The model under review builds one solid part; all positions refer to its coordinate system, in mm. A direction names the side the tool comes from. Round coordinates to 2 decimals unless told otherwise and drop trailing zeros. Write each loop counter-clockwise with the first axis right and the second up, starting at its lowest first coordinate (ties: lowest second). Pieces come first, ordered by that corner, then holes.
Item 1: Draft analysis for pull direction Y (two halves, no side actions). For faces 1 (the face through (-68.862, -31.992, -1.479)), 2 (the face through (55, -21.319, 19)), 3 (the face through (-51.785, 7, 60)), 4 (the face through (-5.215, -16, 48)), state which applies: +Y half, -Y half, draft (parallel to the pull), parting line (faces both ways), or undercut.
Item 2: Add section D-D (y = -3). Give the boundary of the cut face in (x, z) (3 decimals), plus the area to 3 significant figures.
Item 3: Clearance check with flat-ended pins moving along their axes: pin 1 Ø5 at (x, z) = (-39.5, 83.5) entering from +Y; pin 2 Ø5 at (y, z) = (33.5, 116) entering from +X (3 decimals); pin 3 Ø14 at (y, z) = (2.5, 96.5) entering from -X (3 decimals). State where each tip first meets the part, or that it passes through.
Item 4: Add section C-C (z = 118). Give the boundary of the cut face in (x, y) (3 decimals), plus the area to 3 significant figures.
Item 5: Add section B-B (z = 20). Give the boundary of the cut face in (x, y) (3 decimals).
Item 6: To check wall thickness, follow L1, parallel to X at y = 3, z = 41 (3 decimals); L2, parallel to Z at x = 0, y = 26.95; L3, parallel to X at y = 26.5, z = 64 (3 decimals). State the ranges of each line that lie inside material, in increasing order.
Item 7: Machinability: for faces 5 (the face through (57.785, 10, 63)), 6 (the face through (-0.976, 28.116, 27.436)), 7 (the face through (-1, 5, 0)), 8 (the face through (-55, -21.319, 19)), which of the approach directions +Z, -Z, +X, -X, +Y, -Y give a long, thin tool a straight path to every point of the face, cutting with its end or side? Answer none if there is none.
```python
from build123d import *

# Parameters (mm, degrees)
SKETCH001_W     = 145.57
SKETCH001_H     = 82.477117
SKETCH001_R     = 2.185
PAD_DEPTH       = 3
PAD001_DEPTH    = 165.3
SKETCH004_W     = 328.820023
SKETCH004_H     = 275.658927
POCKET_DEPTH    = 200
PAD002_DEPTH    = 3
SKETCH003_R     = 1.4
PAD003_DEPTH    = 10
SKETCH005_R     = 7.5
POCKET001_DEPTH = 46.158923


with BuildPart() as part:
    # Sketch001 → Pad (new body)
    with BuildSketch(Plane.XY):
        with Locations((0, 4.919365)):
            Rectangle(SKETCH001_W, SKETCH001_H)
        with Locations((-67.128146, 40.501069)):
            Circle(SKETCH001_R, mode=Mode.SUBTRACT)
        with Locations((67.128146, 40.501069)):
            Circle(SKETCH001_R, mode=Mode.SUBTRACT)
        with Locations((67.128146, -30.66234)):
            Circle(SKETCH001_R, mode=Mode.SUBTRACT)
        with Locations((-67.128146, -30.66234)):
            Circle(SKETCH001_R, mode=Mode.SUBTRACT)
    extrude(amount=-PAD_DEPTH)

    # Sketch → Pad001 (join)
    with BuildSketch(Plane.XY):
        Polygon((51.785, -21.319194), (57.785, -21.319194), (57.785, 31.157923), (-57.785, 31.157923), (-57.785, -21.319194), (-51.785, -21.319194), (-51.785, 25.157923), (51.785, 25.157923), align=None)
    extrude(amount=PAD001_DEPTH)

    # Sketch004 (on DatumPlane) → Pocket (cut)
    with BuildSketch(Plane(origin=(0, -35, 0), x_dir=(1, 0, 0), z_dir=(0, -0.939693, 0.34202))):
        with Locations((-2.626228, 137.829464)):
            Rectangle(SKETCH004_W, SKETCH004_H)
    extrude(amount=POCKET_DEPTH, mode=Mode.SUBTRACT)

    # Sketch002 (on DatumPlane) → Pad002 (join)
    with BuildSketch(Plane(origin=(0, -35, 0), x_dir=(1, 0, 0), z_dir=(0, -0.939693, 0.34202))):
        Polygon((-57.785, 175.89), (57.785, 175.89), (57.785, 40), (51.785, 40), (51.785, 62), (-5.215, 62), (-5.215, 40), (-57.785, 40), align=None)
    extrude(amount=-PAD002_DEPTH)

    # Sketch003 (on DatumPlane) → Pad003 (join)
    with BuildSketch(Plane(origin=(0, -35, 0), x_dir=(1, 0, 0), z_dir=(0, -0.939693, 0.34202))):
        with Locations((-54.61, 172.715)):
            Circle(SKETCH003_R)
        with Locations((54.61, 172.715)):
            Circle(SKETCH003_R)
        with Locations((54.61, 43.175)):
            Circle(SKETCH003_R)
        with Locations((-54.61, 43.175)):
            Circle(SKETCH003_R)
    extrude(amount=PAD003_DEPTH)

    # Sketch005 → Pocket001 (cut, through all)
    with BuildSketch(Plane.XZ):
        with Locations((0, 20)):
            Circle(SKETCH005_R)
    extrude(amount=-POCKET001_DEPTH, mode=Mode.SUBTRACT)


solid = part.part
```
Numbers:
1. face 1: undercut
1. face 2: -Y half
1. face 3: undercut
1. face 4: draft
2. outline: (-72.785, -3) - (72.785, -3) - (72.785, 0) - (57.785, 0) - (57.785, 87.919) - (-57.785, 87.919) - (-57.785, 0) - (-72.785, 0) - close; hole (-51.785, 0) - (51.785, 0) - (51.785, 79.148) - (-51.785, 79.148) - close
2. area: 2,400 mm2
3. pin 1: stops at y = 31.16
3. pin 2: stops at x = 57.785
3. pin 3: stops at x = -57.785
4. outline: (-57.785, 7.948) - (57.785, 7.948) - (57.785, 31.158) - (-57.785, 31.158) - close; hole (-51.785, 11.141) - (51.785, 11.141) - (51.785, 25.158) - (-51.785, 25.158) - close
4. area: 1,230 mm2
5. outline: (-57.785, -21.319) - (-51.785, -21.319) - (-51.785, 25.158) - (-7.5, 25.158) - (-7.5, 31.158) - (-57.785, 31.158) - close; (7.5, 25.158) - (51.785, 25.158) - (51.785, -21.319) - (57.785, -21.319) - (57.785, 31.158) - (7.5, 31.158) - close
6. L1: x = -57.785 to -51.785, 51.785 to 57.785
6. L2: z = -3 to 12.5, 27.5 to 165.3
6. L3: x = -57.785 to 57.785
7. face 5: +Z, +X, +Y, -Y
7. face 6: +Y, -Y
7. face 7: none
7. face 8: +X, -X, -Y
